Design review of the part built by this model. Coordinates are the model's own, in mm. A direction names the side the tool comes from. Give positions to 0.01 mm unless a question says otherwise; leave off trailing zeros. Order: outer loops, then holes, each group sorted by start corner. A loop starts at its lowest first (then second) coordinate and runs counter-clockwise, first axis right, second up. Notation, with made-up numbers: (36, 30.5) -> (85, 30.5) arc R27 cw to (85, 69.5) -> close; hole circle Ø4 at (80.5, 69.5). An arc over 180 degrees is marked (long way). Return JSON: item names as keys, results as strings.
```python
from build123d import *

# Parameters (mm, degrees)
BOSS_EXTRUDE1_DEPTH      = 4
CHAMFER2_SIZE            = 4
CHAMFER2_OF_MIRROR1_SIZE = 4
SKETCH2_W                = 4
SKETCH2_H                = 4
SKETCH2_W_2              = 8
BOSS_EXTRUDE2_DEPTH      = 4


with BuildPart() as part:
    # Sketch1 → Boss-Extrude1 (new body)
    with BuildSketch(Plane.XY):
        Polygon((0, 0), (0, 30), (-20.5, 30), (-20.5, 24), (-22.5, 24), (-22.5, 18), (-7.5, 18), (-7.5, -4), (-1, -4), (-1, 0), align=None)
    boss_extrude1 = extrude(amount=BOSS_EXTRUDE1_DEPTH)

    # Chamfer2
    chamfer2_edges = [part.edges().sort_by_distance(p)[0] for p in [
        (-7.5, 18, 2),
    ]]
    chamfer(chamfer2_edges, length=CHAMFER2_SIZE)

    # Mirror1: Boss-Extrude1 across plane
    add(boss_extrude1.mirror(Plane(origin=(-22.5, 24, 4), x_dir=(0, 0, 1), z_dir=(1, 0, 0))))

    # Chamfer2 of Mirror1
    chamfer2_of_mirror1_edges = [part.edges().sort_by_distance(p)[0] for p in [
        (-37.5, 18, 2),
    ]]
    chamfer(chamfer2_of_mirror1_edges, length=CHAMFER2_OF_MIRROR1_SIZE)

    # Sketch2 → Boss-Extrude2 (add)
    with BuildSketch(Plane.XY.offset(4)):
        with Locations((-26.5, 32)):
            Rectangle(SKETCH2_W, SKETCH2_H)
        with Locations((-18.5, 32)):
            Rectangle(SKETCH2_W, SKETCH2_H)
        with Locations((-4, 32)):
            Rectangle(SKETCH2_W_2, SKETCH2_H)
        with Locations((-41, 32)):
            Rectangle(SKETCH2_W_2, SKETCH2_H)
    extrude(amount=-BOSS_EXTRUDE2_DEPTH)


solid = part.part
```
Item 1: For pin 1 (5 mm diameter, centred on x = -33, y = 11, fed in from +Z); pin 2 (1.2 mm diameter, centred on y = -2.5, z = 2, fed in from -X); pin 3 (2 mm diameter, centred on x = -23, z = 1, fed in from +Y); pin 4 (2 mm diameter, centred on x = -12, z = 1.5, fed in from +Y), all flat-tipped, find the tip position at first contact; note any pin that passes through.
Result set:
{"pin 1": "passes through", "pin 2": "stops at x = -44", "pin 3": "stops at y = 24", "pin 4": "stops at y = 30"}
Item 2: Add section C-C (z = 1.65). Give the boundary of the cut face in (x, y).
Result set:
{"outline": "(-45, 0) -> (-44, 0) -> (-44, -4) -> (-37.5, -4) -> (-37.5, 14) -> (-33.5, 18) -> (-11.5, 18) -> (-7.5, 14) -> (-7.5, -4) -> (-1, -4) -> (-1, 0) -> (0, 0) -> (0, 34) -> (-8, 34) -> (-8, 30) -> (-16.5, 30) -> (-16.5, 34) -> (-20.5, 34) -> (-20.5, 24) -> (-24.5, 24) -> (-24.5, 34) -> (-28.5, 34) -> (-28.5, 30) -> (-37, 30) -> (-37, 34) -> (-45, 34) -> close"}
Item 3: Mouldability with a two-part tool opening along X and no side actions: class faces 1 (the face through (-16.5, 32, 2)), 2 (the face through (-4, -4, 2)), 3 (the face through (-45, 17, 2)), 4 (the face through (-12, 30, 2)) as released by +X, released by -X, zero draft, split by the parting line, or undercut.
Result set:
{"face 1": "undercut", "face 2": "zero draft", "face 3": "released by -X", "face 4": "undercut"}
Item 4: Add section D-D (y = 25). Give the boundary of the cut face in (x, z).
Result set:
{"outline": "(-45, 0) -> (-24.5, 0) -> (-24.5, 4) -> (-45, 4) -> close; (-20.5, 0) -> (0, 0) -> (0, 4) -> (-20.5, 4) -> close"}
Item 5: Add section A-A (y = 5.5). Give the boundary of the cut face in (x, z).
Result set:
{"outline": "(-45, 0) -> (-37.5, 0) -> (-37.5, 4) -> (-45, 4) -> close; (-7.5, 0) -> (0, 0) -> (0, 4) -> (-7.5, 4) -> close"}
Item 6: Add section B-B (y = 31). Give the boundary of the cut face in (x, z).
Result set:
{"outline": "(-45, 0) -> (-37, 0) -> (-37, 4) -> (-45, 4) -> close; (-28.5, 0) -> (-24.5, 0) -> (-24.5, 4) -> (-28.5, 4) -> close; (-20.5, 0) -> (-16.5, 0) -> (-16.5, 4) -> (-20.5, 4) -> close; (-8, 0) -> (0, 0) -> (0, 4) -> (-8, 4) -> close"}
Item 7: Machinability: for faces 5 (the face through (-33, 30, 2)), 6 (the face through (-22, 18, 2)), 7 (the face through (-44.5, 0, 2)), which of the approach directions +Z, -Z, +X, -X, +Y, -Y give a long, thin tool a straight path to every point of the face, cutting with its end or side? Answer none if there is none.
Result set:
{"face 5": "+Z, -Z, +Y", "face 6": "+Z, -Z, -Y", "face 7": "+Z, -Z, -X, -Y"}
Item 8: Wall thickness on L1, parallel to X at y = 31, z = 0.3; L2, parallel to X at y = 2, z = 3.4; L3, parallel to X at y = 26.5, z = 2.15: over which ranges is each line inside the solid? List them lowest first. Write a range as [from, to].
Result set:
{"L1": "x = [-45, -37], [-28.5, -24.5], [-20.5, -16.5], [-8, 0]", "L2": "x = [-45, -37.5], [-7.5, 0]", "L3": "x = [-45, -24.5], [-20.5, 0]"}
